The model under review builds one solid part; all positions refer to its coordinate system, in mm. Face numbers are marked on the shaded views. A direction names the side the tool comes from. Round coordinates to 2 decimals unless told otherwise and drop trailing zeros. Write each loop counter-clockwise with the first axis right and the second up, starting at its lowest first coordinate (ties: lowest second). Pieces come first, ordered by that corner, then holes.
Item 1: Add section D-D (y = 10). Give the boundary of the cut face in (x, z).
Item 2: Clearance check with a flat-ended pin moving along its axis: pin 1 Ø5 at (y, z) = (27, 18) entering from -X. State where the tip first meets the part, or that it passes through.
Item 3: Add section C-C (z = 7.5). Give the boundary of the cut face in (x, y).
Item 4: Add section A-A (x = 25). Give the boundary of the cut face in (y, z), plus the area to 3 significant figures.
Item 5: Add section B-B (y = 35). Give the boundary of the cut face in (x, z), plus the area to 3 significant figures.
Item 6: Draft analysis for pull direction Z (two halves, no side actions). For the marked faces 1, 2 and 3, state which applies: +Z half, -Z half, draft (parallel to the pull), parting line (faces both ways), or undercut.
Item 7: Machinability: for the marked faces 4 and 5, which of the approach directions +Z, -Z, +X, -X, +Y, -Y give a long, thin tool a straight path to every point of the face, cutting with its end or side? Answer none if there is none.
Item 8: To check wall thickness, follow L1, parallel to Z at x = 5.5, y = 36; L2, parallel to Y at x = 25, z = 3; L3, parallel to Z at x = 3, y = 8. State the ranges of each line that lie inside material, in increasing order.
```python
from build123d import *

# Parameters (mm, degrees)
ESBO_O1_W                = 50
ESBO_O1_H                = 50
RESSALTO_EXTRUS_O1_DEPTH = 55
CASCA2_T                 = -5
ESBO_O2_R                = 2.25
CORTE_EXTRUS_O1_DEPTH    = 90.582364336
ESBO_O3_W                = 10
ESBO_O3_H                = 45
CORTE_EXTRUS_O2_DEPTH    = 90.582364336


with BuildPart() as part:
    # Esboço1 → Ressalto-extrusão1 (new body)
    with BuildSketch(Plane.XY):
        with Locations((25, 25)):
            Rectangle(ESBO_O1_W, ESBO_O1_H)
    extrude(amount=RESSALTO_EXTRUS_O1_DEPTH)

    # Casca2
    casca2_openings = [part.faces().sort_by_distance(p)[0] for p in [
        (25, 0, 27.5),
    ]]
    offset(amount=CASCA2_T, openings=casca2_openings, kind=Kind.INTERSECTION)

    # Esboço2 → Corte-extrusão1 (cut, through all)
    with BuildSketch(Plane.XY.offset(55)):
        with Locations((25, 10)):
            Circle(ESBO_O2_R)
    extrude(amount=-CORTE_EXTRUS_O1_DEPTH, mode=Mode.SUBTRACT)

    # Esboço3 → Corte-extrusão2 (cut, through all)
    with BuildSketch(Plane(origin=(50, 0, 0), x_dir=(0, 0, -1), z_dir=(1, 0, 0))):
        with Locations((-27.5, 22.5)):
            Rectangle(ESBO_O3_W, ESBO_O3_H)
    extrude(amount=-CORTE_EXTRUS_O2_DEPTH, mode=Mode.SUBTRACT)


solid = part.part
```
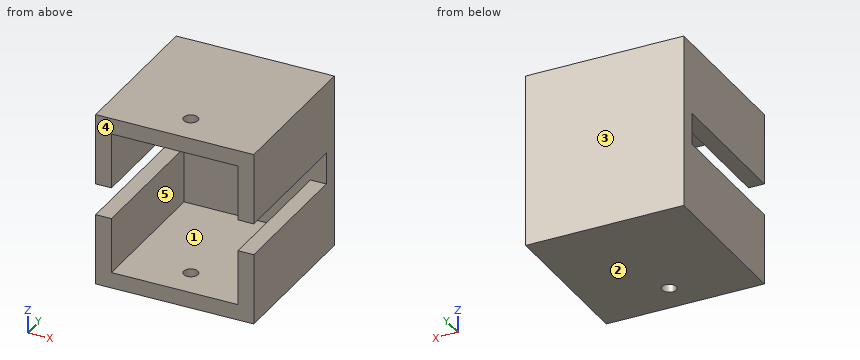
Numbers:
1. outline: (0, 0) - (22.75, 0) - (22.75, 5) - (5, 5) - (5, 22.5) - (0, 22.5) - close; (0, 32.5) - (5, 32.5) - (5, 50) - (22.75, 50) - (22.75, 55) - (0, 55) - close; (27.25, 0) - (50, 0) - (50, 22.5) - (45, 22.5) - (45, 5) - (27.25, 5) - close; (27.25, 50) - (45, 50) - (45, 32.5) - (50, 32.5) - (50, 55) - (27.25, 55) - close
2. pin 1: stops at x = 0
3. outline: (0, 0) - (5, 0) - (5, 45) - (45, 45) - (45, 0) - (50, 0) - (50, 50) - (0, 50) - close
4. outline: (0, 0) - (7.75, 0) - (7.75, 5) - (0, 5) - close; (0, 50) - (7.75, 50) - (7.75, 55) - (0, 55) - close; (12.25, 0) - (50, 0) - (50, 55) - (12.25, 55) - (12.25, 50) - (45, 50) - (45, 5) - (12.25, 5) - close
4. area: 680 mm2
5. outline: (0, 0) - (50, 0) - (50, 22.5) - (45, 22.5) - (45, 5) - (5, 5) - (5, 22.5) - (0, 22.5) - close; (0, 32.5) - (5, 32.5) - (5, 50) - (45, 50) - (45, 32.5) - (50, 32.5) - (50, 55) - (0, 55) - close
5. area: 850 mm2
6. face 1: undercut
6. face 2: -Z half
6. face 3: draft
7. face 4: +Z, -Z, +X, -X, -Y
7. face 5: -Y
8. L1: z = 0 to 5, 50 to 55
8. L2: y = 0 to 7.75, 12.25 to 50
8. L3: z = 0 to 22.5, 32.5 to 55
